```python
from build123d import *

# Parameters (mm, degrees)
SKETCH1_W               = 35
SKETCH1_H               = 20
BOSS_EXTRUDE1_DEPTH     = 45
SKETCH2_R               = 7.75
CUT_EXTRUDE1_DEPTH      = 46
SKETCH3_R               = 4.25
CUT_EXTRUDE2_DEPTH      = 10
SKETCH4_W               = 25
SKETCH4_H               = 15
BOSS_EXTRUDE2_DEPTH     = 25
SKETCH5_W               = 14.5
SKETCH5_H               = 16.25
CUT_EXTRUDE3_DEPTH      = 31
BOSS_EXTRUDE3_REACH     = 31.75
SKETCH6_W               = 16.25
SKETCH6_H               = 3.25
SKETCH7_R               = 5.25
CUT_EXTRUDE4_DEPTH      = 27.75
CUT_EXTRUDE4_DEPTH_BACK = 19.25
CHAMFER1_SIZE           = 1
CHAMFER2_SIZE           = 1


with BuildPart() as part:
    # Sketch1 → Boss-Extrude1 (new body)
    with BuildSketch(Plane(origin=(0, 0, 0), x_dir=(1, 0, 0), z_dir=(0, 1, 0))):
        with Locations((17.5, 10)):
            Rectangle(SKETCH1_W, SKETCH1_H)
    extrude(amount=BOSS_EXTRUDE1_DEPTH)

    # Sketch2 → Cut-Extrude1 (cut, through all)
    with BuildSketch(Plane(origin=(0, 45, 0), x_dir=(1, 0, 0), z_dir=(0, 1, 0))):
        with Locations((10, 10)):
            Circle(SKETCH2_R)
    extrude(amount=-CUT_EXTRUDE1_DEPTH, mode=Mode.SUBTRACT)

    # Sketch3 → Cut-Extrude2 (cut)
    with BuildSketch(Plane(origin=(35, 0, 0), x_dir=(0, 0, -1), z_dir=(1, 0, 0))):
        with Locations((10, 37.6875)):
            Circle(SKETCH3_R)
        with Locations((10, 7.3125)):
            Circle(SKETCH3_R)
    extrude(amount=-CUT_EXTRUDE2_DEPTH, mode=Mode.SUBTRACT)

    # Sketch4 → Boss-Extrude2 (add)
    with BuildSketch(Plane(origin=(0, 0, -20), x_dir=(-1, 0, 0), z_dir=(0, 0, -1))):
        with Locations((-12.5, 22.5)):
            Rectangle(SKETCH4_W, SKETCH4_H)
    extrude(amount=BOSS_EXTRUDE2_DEPTH)

    # Sketch5 → Cut-Extrude3 (cut, through all)
    with BuildSketch(Plane(origin=(0, 30, 0), x_dir=(1, 0, 0), z_dir=(0, 1, 0))):
        with Locations((12.5, 36.875)):
            Rectangle(SKETCH5_W, SKETCH5_H)
    extrude(amount=-CUT_EXTRUDE3_DEPTH, mode=Mode.SUBTRACT)

    # Sketch6 → Boss-Extrude3 (add, up to next)
    with BuildSketch(Plane(origin=(5.25, 0, 0), x_dir=(0, 0, -1), z_dir=(1, 0, 0)), mode=Mode.PRIVATE) as boss_extrude3_sk1:
        with Locations((36.875, 28.375)):
            Rectangle(SKETCH6_W, SKETCH6_H)
    boss_extrude3_tool1 = extrude(boss_extrude3_sk1.sketch, amount=BOSS_EXTRUDE3_REACH, mode=Mode.PRIVATE) - part.part
    add(boss_extrude3_tool1.solids().sort_by_distance((5.25, 28.375, -36.875))[0])
    # Sketch6 → Boss-Extrude3 (add, up to next)
    with BuildSketch(Plane(origin=(5.25, 0, 0), x_dir=(0, 0, -1), z_dir=(1, 0, 0)), mode=Mode.PRIVATE) as boss_extrude3_sk2:
        with Locations((36.875, 16.625)):
            Rectangle(SKETCH6_W, SKETCH6_H)
    boss_extrude3_tool2 = extrude(boss_extrude3_sk2.sketch, amount=BOSS_EXTRUDE3_REACH, mode=Mode.PRIVATE) - part.part
    add(boss_extrude3_tool2.solids().sort_by_distance((5.25, 16.625, -36.875))[0])

    # Sketch7 → Cut-Extrude4 (cut, two sides)
    with BuildSketch(Plane(origin=(0, 18.25, 0), x_dir=(1, 0, 0), z_dir=(0, 1, 0))) as cut_extrude4_sk:
        with Locations((12.5, 36.917096231)):
            Circle(SKETCH7_R)
    extrude(amount=CUT_EXTRUDE4_DEPTH, mode=Mode.SUBTRACT)
    extrude(cut_extrude4_sk.sketch, amount=-CUT_EXTRUDE4_DEPTH_BACK, mode=Mode.SUBTRACT)

    # Chamfer1
    chamfer1_edges = [part.edges().sort_by_distance(p)[0] for p in [
        (35, 45, -10),
        (2.25, 0, -10),
        (2.25, 45, -10),
        (17.5, 45, -20),
        (0, 7.5, -20),
        (0, 15, -32.5),
        (12.5, 30, -20),
        (0, 30, -32.5),
        (25, 22.5, -20),
        (25, 30, -32.5),
        (12.5, 15, -20),
        (25, 15, -32.5),
        (0, 22.5, -45),
        (12.5, 30, -45),
        (25, 22.5, -45),
        (12.5, 15, -45),
        (0, 45, -10),
        (17.5, 0, -20),
        (35, 0, -10),
        (17.5, 0, 0),
        (0, 0, -10),
        (0, 37.5, -20),
        (35, 22.5, -20),
        (35, 22.5, 0),
        (0, 22.5, 0),
        (7.25, 26.75, -36.917096231),
        (7.25, 30, -36.917096231),
        (7.25, 18.25, -36.917096231),
        (7.25, 15, -36.917096231),
        (17.5, 45, 0),
    ]]
    chamfer(chamfer1_edges, length=CHAMFER1_SIZE)

    # Chamfer2
    chamfer2_edges = [part.edges().sort_by_distance(p)[0] for p in [
        (35, 37.6875, -5.75),
        (35, 7.3125, -5.75),
    ]]
    chamfer(chamfer2_edges, length=CHAMFER2_SIZE)


solid = part.part
```
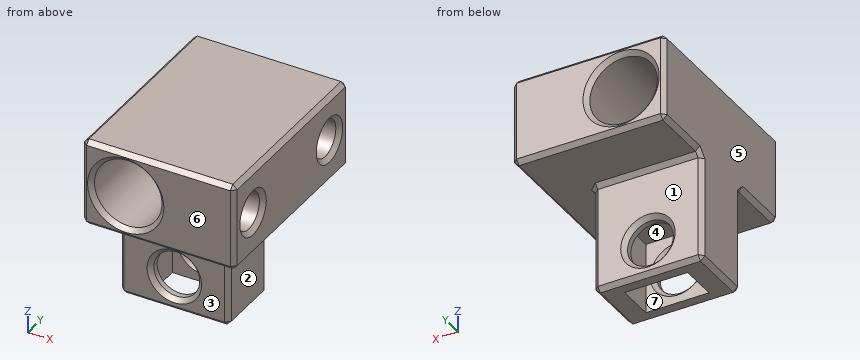
Could you check a few things on this model? Use its own coordinates, in mm. Face numbers are marked on the shaded views. A direction names the side the tool comes from. Coordinates: 2 decimals unless noted, no trailing zeros. Write each loop counter-clockwise with the first axis right and the second up, starting at its lowest first coordinate (ties: lowest second). Pieces come first, ordered by that corner, then holes. Notation, with made-up numbers: (-30.75, -14) -> (12.25, -14) arc R15 cw to (12.25, 9) -> close; hole circle Ø11 at (49, 27). An arc over 180 degrees is marked (long way). One line per question, with ' | ' between items. Start each with the question number.
1. Will these pins go through, and if not, where does the flat tip stop? P1, Ø4.5, axis at x = 15.5, z = -33, coming from the -Y side; P2, Ø4, axis at y = 20, z = -33, coming from the +X side; P3, Ø4, axis at y = 10, z = -8.5, coming from the +X side; P4, Ø7, axis at y = 5.5, z = -11, coming from the +X side.
2. If we section it at C-C (z = -30): Please give me the cut outline in (x, y), and give its area (3 significant figures).
3. For the marked faces 1, 2 and 3, which set-ups out of +Z, -Z, +X, -X, +Y, -Y let a thin tool reach every point of the face, with its end or its side?
4. If we section it at B-B (z = -10): Please give me the cut outline in (x, y).
5. Thinking about a two-plate mould opening in Y: for the marked faces 4, 5, 6 and 7, which applies, pulls with the +Y half, pulls with the -Y half, needs draft (parallel to the pull), parting line crosses it, or undercut?
6. If we section it at A-A (y = 22): Please give me the cut outline in (x, z).
7. If we section it at D-D (x = 29): Please give me the cut outline in (y, z), and give its area (3 significant figures).
8. Please list where these lines run through material, in increasing order: line 1 along Z through (x, y) = (10, 32); line 2 along Y through (x, z) = (31, -10); line 3 along Z through (x, y) = (10, 16).
Return value:
1) P1: stops at y = 15 | P2: stops at x = 25 | P3: stops at x = 34.83 | P4: stops at x = 35
2) outline: (0, 16) -> (1, 15) -> (24, 15) -> (25, 16) -> (25, 29) -> (24, 30) -> (1, 30) -> (0, 29) -> close; hole (5.25, 18.25) -> (19.75, 18.25) -> (19.75, 26.75) -> (5.25, 26.75) -> close | area: 250 mm²
3) face 1: -Z, +X, -X, +Y | face 2: -Z, +X, +Y, -Y | face 3: -Z, +X, -X, -Y
4) outline: (0, 1) -> (1, 0) -> (1.25, 0) -> (2.25, 1) -> (2.25, 44) -> (1.25, 45) -> (1, 45) -> (0, 44) -> close; (17.75, 1) -> (18.75, 0) -> (34, 0) -> (35, 1) -> (35, 2.06) -> (34, 3.06) -> (25, 3.06) -> (25, 11.56) -> (34, 11.56) -> (35, 12.56) -> (35, 32.44) -> (34, 33.44) -> (25, 33.44) -> (25, 41.94) -> (34, 41.94) -> (35, 42.94) -> (35, 44) -> (34, 45) -> (18.75, 45) -> (17.75, 44) -> close
5) face 4: undercut | face 5: needs draft | face 6: pulls with the -Y half | face 7: undercut
6) outline: (0, -44) -> (1, -45) -> (5.25, -45) -> (5.25, -28.75) -> (19.75, -28.75) -> (19.75, -45) -> (24, -45) -> (25, -44) -> (25, -21) -> (26, -20) -> (34, -20) -> (35, -19) -> (35, -1) -> (34, 0) -> (1, 0) -> (0, -1) -> close; hole circle Ø15.5 at (10, -10)
7) outline: (0, -19) -> (1, -20) -> (44, -20) -> (45, -19) -> (45, -1) -> (44, 0) -> (1, 0) -> (0, -1) -> close; hole circle Ø8.5 at (7.31, -10); hole circle Ø8.5 at (37.69, -10) | area: 785 mm²
8) line 1: z = -20 to -17.75, -2.25 to 0 | line 2: y = 0 to 3.06, 11.56 to 33.44, 41.94 to 45 | line 3: z = -45 to -41.53, -32.3 to -17.75, -2.25 to 0
